Answer from the drawing. Dimensions are ordinates in mm from the lowest x, y and z of the part. Give positions to 0.01 mm unless a question says otherwise; leave off trailing zeros. Loops run counter-clockwise (first coordinate to the right, second up) from the corner with the lowest first, then second, coordinate; pieces in that order, holes last. Notation, with made-up numbers: (37.25, -26.75) - (44.25, -26.75) arc R15 ccw to (44.25, -13.75) - close; hole circle Ø4 at (-33.75, 82). An arc over 180 degrees is marked (long way). Put each result on its own line as item: value. Start each with the question number.
1. Consider L1, parallel to Y at x = 34, z = 26; L2, parallel to Y at x = 22, z = 19.5; L3, parallel to X at y = 30.5, z = 34. Determine where each line is inside the solid, lowest interval first. Write a range as from..to.
2. A cutting plane is placed at A-A, the plane x = 34. Determine the outline of the cut face in (y, z), plus the area to 3 significant figures.
3. For a pull along X with two mould halves and no side action, classify the marked faces 1, 2 and 3 as released by +X, released by -X, zero draft, split by the parting line, or undercut.
4. A cutting plane is placed at C-C, the plane z = 15. Determine the outline of the cut face in (x, y).
5. Given pin 1 Ø2 at (x, z) = (17, 26.5) entering from -Y; pin 2 Ø2.5 at (x, z) = (36, 19.5) entering from -Y; pin 3 Ø3 at (y, z) = (51, 26) entering from -X, each flat-ended and moving along its own axis, determine where each tip first touches the part or whether it passes through.
6. A cutting plane is placed at D-D, the plane y = 62.5. Determine the outline of the cut face in (x, z), plus the area to 3 significant figures.
7. A cutting plane is placed at B-B, the plane y = 34. Determine the outline of the cut face in (x, z).
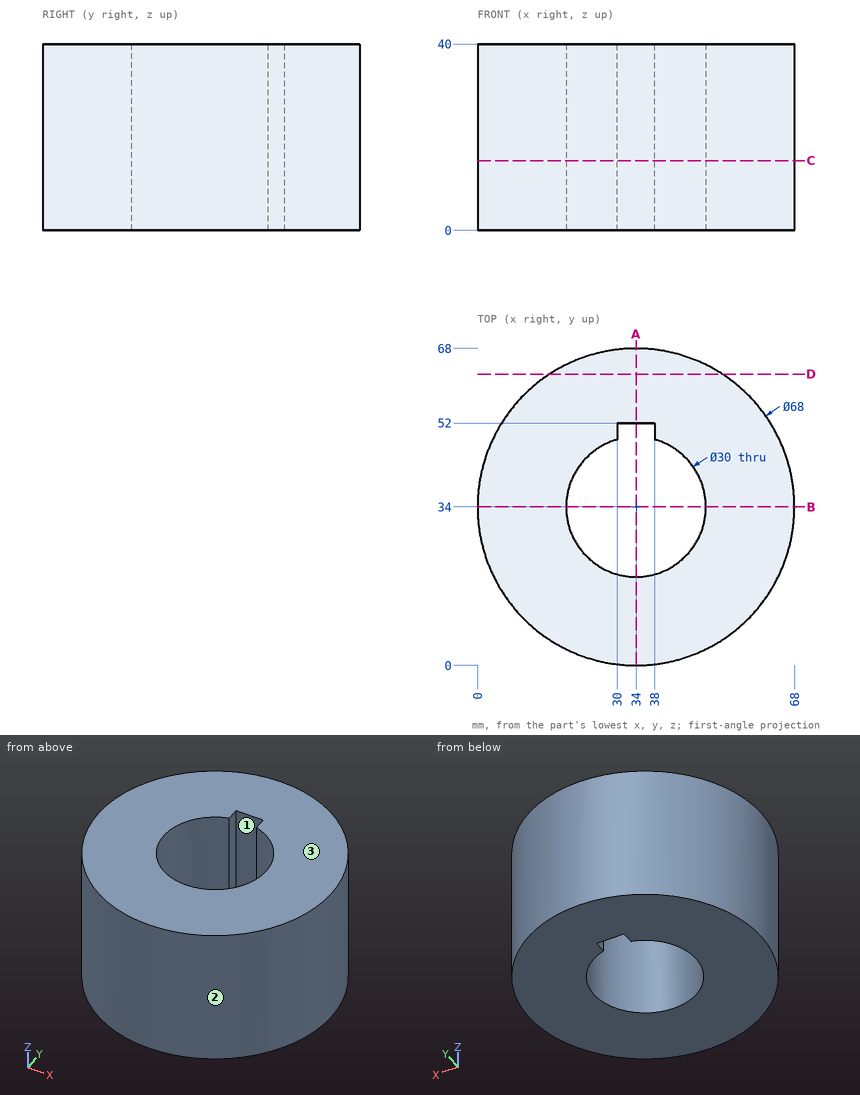
Return value:
1. L1: y = 0..19, 52..68
1. L2: y = 2.19..25, 43..65.81
1. L3: x = 0.18..19.41, 48.59..67.82
2. outline: (0, 0) - (19, 0) - (19, 40) - (0, 40) - close; (52, 0) - (68, 0) - (68, 40) - (52, 40) - close
2. area: 1,400 mm2
3. face 1: undercut
3. face 2: split by the parting line
3. face 3: zero draft
4. outline: circle Ø68 at (34, 34); hole (30, 48.46) arc R15 ccw (long way) to (38, 48.46) - (38, 52) - (30, 52) - close
5. pin 1: stops at y = 4
5. pin 2: stops at y = 0.01
5. pin 3: stops at x = 3.74
6. outline: (15.46, 0) - (52.54, 0) - (52.54, 40) - (15.46, 40) - close
6. area: 1,480 mm2
7. outline: (0, 0) - (19, 0) - (19, 40) - (0, 40) - close; (49, 0) - (68, 0) - (68, 40) - (49, 40) - close
